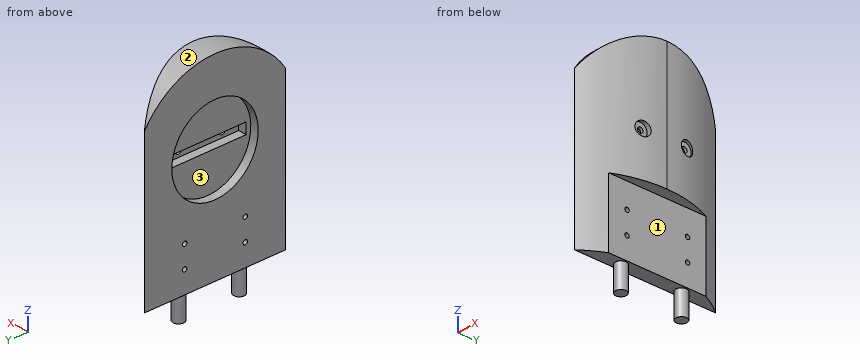
```python
from build123d import *

# Parameters (mm, degrees)
SKETCH_1_W          = 9
SKETCH_1_H          = 60
EXTRUDE_1_DEPTH     = 41.2
SKETCH_4_R          = 30
EXTRUDE_3_DEPTH     = 9
CUT_EXTRUDE_1_DEPTH = 72
SKETCH_5_R          = 15.7
CUT_EXTRUDE_2_DEPTH = 3
SKETCH_6_W          = 4
SKETCH_6_H          = 28
CUT_EXTRUDE_3_DEPTH = 3
SKETCH_7_R          = 2
EXTRUDE_4_DEPTH     = 9
SKETCH_8_W          = 4
SKETCH_8_H          = 82.4
CUT_EXTRUDE_4_DEPTH = 25
SKETCH_9_R          = 0.8
CUT_EXTRUDE_5_DEPTH = 5
SKETCH_10_R         = 1
CUT_EXTRUDE_6_DEPTH = 1
SKETCH_11_R         = 2.5
CUT_EXTRUDE_7_DEPTH = 3


with BuildPart() as part:
    # 草图1 → 凸台-拉伸1 (new body)
    with BuildSketch(Plane.XY):
        with Locations((36.7, 0)):
            Rectangle(SKETCH_1_W, SKETCH_1_H)
    extrude(amount=EXTRUDE_1_DEPTH)

    # 草图4 → 凸台-拉伸3 (add)
    with BuildSketch(Plane.ZY.offset(-32.2)):
        with Locations((41.2, 0)):
            Circle(SKETCH_4_R)
    extrude(amount=-EXTRUDE_3_DEPTH)

    # 切除-拉伸1: read off the stored shape, not the designer's step
    # 切除-拉伸1 outline → 切除-拉伸1 (cut)
    with BuildSketch(Plane.XY):
        with BuildLine():
            Line((32.2, 30), (32.2, 25.702139989))
            ThreePointArc((32.2, 25.702139989), (38.884958532, 13.616166862), (41.2, 0))
            Line((41.2, 0), (41.2, 30))
            Line((41.2, 30), (32.2, 30))
        make_face()
        with BuildLine():
            Line((41.2, -30), (41.2, 0))
            ThreePointArc((41.2, 0), (38.884958532, -13.616166862), (32.2, -25.702139989))
            Line((32.2, -25.702139989), (32.2, -30))
            Line((32.2, -30), (41.2, -30))
        make_face()
    extrude(amount=CUT_EXTRUDE_1_DEPTH, mode=Mode.SUBTRACT)

    # 草图5 → 切除-拉伸2 (cut)
    with BuildSketch(Plane.ZY.offset(-32.2)):
        with Locations((41.2, 0)):
            Circle(SKETCH_5_R)
    extrude(amount=-CUT_EXTRUDE_2_DEPTH, mode=Mode.SUBTRACT)

    # 草图6 → 切除-拉伸3 (cut)
    with BuildSketch(Plane.ZY.offset(-35.2)):
        with Locations((41.2, 0)):
            Rectangle(SKETCH_6_W, SKETCH_6_H)
    extrude(amount=-CUT_EXTRUDE_3_DEPTH, mode=Mode.SUBTRACT)

    # 草图7 → 凸台-拉伸4 (add)
    with BuildSketch(Plane(origin=(0, 0, 0), x_dir=(-1, 0, 0), z_dir=(0, 0, -1))):
        with Locations(Location((-34.7, 11, 0), (0, 0, 180))):
            Circle(SKETCH_7_R)
        with Locations(Location((-34.7, -11, 0), (0, 0, 180))):
            Circle(SKETCH_7_R)
    extrude(amount=EXTRUDE_4_DEPTH)

    # 草图8 → 切除-拉伸4 (cut)
    with BuildSketch(Plane.XY):
        with Locations((39.2, 0)):
            Rectangle(SKETCH_8_W, SKETCH_8_H)
    extrude(amount=CUT_EXTRUDE_4_DEPTH, mode=Mode.SUBTRACT)

    # 草图9 → 切除-拉伸5 (cut)
    with BuildSketch(Plane(origin=(37.2, 0, 0), x_dir=(0, 0, -1), z_dir=(1, 0, 0))):
        with Locations((-16, -11)):
            Circle(SKETCH_9_R)
        with Locations((-8, -11)):
            Circle(SKETCH_9_R)
        with Locations((-16, 11)):
            Circle(SKETCH_9_R)
        with Locations((-8, 11)):
            Circle(SKETCH_9_R)
    extrude(amount=-CUT_EXTRUDE_5_DEPTH, mode=Mode.SUBTRACT)

    # 草图10 → 切除-拉伸6 (cut)
    with BuildSketch(Plane.ZY.offset(-38.2)):
        with Locations((41.2, 8)):
            Circle(SKETCH_10_R)
        with Locations((41.2, -8)):
            Circle(SKETCH_10_R)
    extrude(amount=-CUT_EXTRUDE_6_DEPTH, mode=Mode.SUBTRACT)

    # 草图11 → 切除-拉伸7 (cut)
    with BuildSketch(Plane.ZY.offset(-39.2)):
        with Locations((41.2, 8)):
            Circle(SKETCH_11_R)
        with Locations((41.2, -8)):
            Circle(SKETCH_11_R)
    extrude(amount=-CUT_EXTRUDE_7_DEPTH, mode=Mode.SUBTRACT)


solid = part.part
```
Input: part model. Units: mm. Frame: model coordinates. Face numbers are marked on the shaded views. Coordinates: 2 decimals unless noted, no trailing zeros. Loops run counter-clockwise (first coordinate to the right, second up) from the corner with the lowest first, then second, coordinate; pieces in that order, holes last. Notation, with made-up numbers: M 65.25,-38 L 91.25,-38 A23 ccw 91.25,-16 Z; hole C 14.25,26 d10. An arc over 180 degrees is marked long. Use a Markdown table: item, result. Add a question column.
1) Draft query along Y for the marked faces 1, 2 and 3. Return one class per face: +Y half, -Y half, draft (parallel to the pull), parting line (faces both ways), or undercut.
2) Pin query (flat end, axial travel): P1, Ø10, axis at y = 4.5, z = 31.5, coming from the +X side; P2, Ø2.5, axis at y = -8, z = 41.2, coming from the +X side; P3, Ø8, axis at y = 8, z = 41.2, coming from the -X side; P4, Ø2.5, axis at y = -11, z = 16, coming from the +X side. Return the tip coordinate at first contact, or that it passes through.
3) Line query: L1, parallel to Y at x = 33.9, z = 8; L2, parallel to Y at x = 34.8, z = 8; L3, parallel to Z at x = 33, y = -10.5. Output: solid intervals per line, ascending. Write a range as from..to.
4) Section D-D, the plane z = 29.5. Return the cut outline in (x, y).
5) Section B-B, the plane y = 8. Return the cut outline in (x, z), plus the area to 3 significant figures.
6) Section A-A, the plane z = 16. Return the cut outline in (x, y), plus the area to 3 significant figures.
7) Section C-C, the plane z = 41.2. Return the cut outline in (x, y), plus the area to 3 significant figures.
Answer below:
| question | item | result |
|---|---|---|
| 1 | face 1 | draft |
| 1 | face 2 | parting line |
| 1 | face 3 | undercut |
| 2 | P1 | x = 41.2 |
| 2 | P2 | x = 39.2 |
| 2 | P3 | x = 35.2 |
| 2 | P4 | x = 37.2 |
| 3 | L1 | -23.41..-11.8, -10.2..10.2, 11.8..23.41 |
| 3 | L2 | -22.05..-11.8, -10.2..10.2, 11.8..22.05 |
| 3 | L3 | -9..7.38, 8.62..15.38, 16.62..29.53, 52.87..69.3 |
| 4 | outline | M 32.2,-25.7 A41.2 ccw 32.2,25.7 L 32.2,10.47 L 35.2,10.47 L 35.2,-10.47 L 32.2,-10.47 Z |
| 5 | outline | M 32.2,0 L 37.2,0 L 37.2,25 L 40.42,25 L 40.42,38.7 L 39.2,38.7 L 39.2,40.2 L 38.2,40.2 L 38.2,39.2 L 35.2,39.2 L 35.2,27.69 L 32.2,27.69 Z; M 32.2,54.71 L 35.2,54.71 L 35.2,43.2 L 38.2,43.2 L 38.2,42.2 L 39.2,42.2 L 39.2,43.7 L 40.42,43.7 L 40.42,70.11 L 32.2,70.11 Z |
| 5 | area | 395 mm2 |
| 6 | outline | M 32.2,-25.7 A41.2 ccw 37.2,-17.71 L 37.2,-11.8 L 32.2,-11.8 Z; M 32.2,-10.2 L 37.2,-10.2 L 37.2,10.2 L 32.2,10.2 Z; M 32.2,11.8 L 37.2,11.8 L 37.2,17.71 A41.2 ccw 32.2,25.7 Z |
| 6 | area | 204 mm2 |
| 7 | outline | M 32.2,-25.7 A41.2 ccw 39.84,-10.5 L 39.2,-10.5 L 39.2,-9 L 38.2,-9 L 38.2,-14 L 35.2,-14 L 35.2,-15.7 L 32.2,-15.7 Z; M 32.2,15.7 L 35.2,15.7 L 35.2,14 L 38.2,14 L 38.2,9 L 39.2,9 L 39.2,10.5 L 39.84,10.5 A41.2 ccw 32.2,25.7 Z; M 38.2,-7 L 39.2,-7 L 39.2,-5.5 L 40.83,-5.5 A41.2 ccw 40.83,5.5 L 39.2,5.5 L 39.2,7 L 38.2,7 Z |
| 7 | area | 122 mm2 |
